Geometry: final body of the model. Coordinates: model frame, mm. Round coordinates to 2 decimals unless told otherwise and drop trailing zeros. Loops run counter-clockwise (first coordinate to the right, second up) from the corner with the lowest first, then second, coordinate; pieces in that order, holes last. Notation, with made-up numbers: (16.25, -27) -> (31.25, -27) arc R16 cw to (31.25, -8) -> close; hole circle Ø4 at (62.25, 22.25). An arc over 180 degrees is marked (long way). Answer in a Markdown table with one row per item.
```python
from build123d import *

# Parameters (mm, degrees)
SKETCH1_R               = 6.35
BOSS_EXTRUDE1_DEPTH     = 531
SKETCH2_R               = 5.5
BOSS_EXTRUDE2_DEPTH     = 2
BOSS_EXTRUDE3_START     = 2
SKETCH3_R               = 5.5
BOSS_EXTRUDE3_DEPTH     = 2
CUT_EXTRUDE1_DEPTH      = 536.075363851
CUT_EXTRUDE1_DEPTH_BACK = 536.075363851
SKETCH4_R               = 2.375


with BuildPart() as part:
    # Sketch1 → Boss-Extrude1 (new body)
    with BuildSketch(Plane.XY):
        Circle(SKETCH1_R)
    extrude(amount=BOSS_EXTRUDE1_DEPTH)

    # Sketch2 → Boss-Extrude2 (add)
    with BuildSketch(Plane.XY.offset(531)):
        Circle(SKETCH2_R)
    extrude(amount=BOSS_EXTRUDE2_DEPTH)

    # Sketch3 → Boss-Extrude3 (add)
    with BuildSketch(Plane(origin=(0, 0, 0), x_dir=(-1, 0, 0), z_dir=(0, 0, -1)).offset(BOSS_EXTRUDE3_START)):
        with Locations(Location((0, 0, 0), (0, 0, 180))):
            Circle(SKETCH3_R)
    extrude(amount=-BOSS_EXTRUDE3_DEPTH)

    # Sketch4 → Cut-Extrude1 (cut, two sides: drawn at the far end of the back side and taken through both)
    with BuildSketch(Plane(origin=(0, 0, -2), x_dir=(-1, 0, 0), z_dir=(0, 0, -1)).offset(-CUT_EXTRUDE1_DEPTH_BACK)):
        Circle(SKETCH4_R)
    extrude(amount=CUT_EXTRUDE1_DEPTH + CUT_EXTRUDE1_DEPTH_BACK, mode=Mode.SUBTRACT)


solid = part.part
```
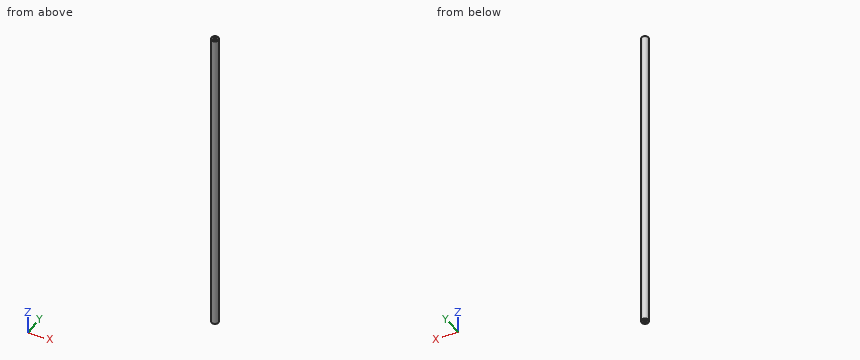
Item 1: Cut plane A-A (y = 0). Output: boundary loops of the cut face in (x, z) (3 decimals).
Answer:
| item | result |
|---|---|
| outline | (-6.35, 0) -> (-5.5, 0) -> (-5.5, -2) -> (-2.375, -2) -> (-2.375, 533) -> (-5.5, 533) -> (-5.5, 531) -> (-6.35, 531) -> close; (2.375, -2) -> (5.5, -2) -> (5.5, 0) -> (6.35, 0) -> (6.35, 531) -> (5.5, 531) -> (5.5, 533) -> (2.375, 533) -> close |
Item 2: Pin query (flat end, axial travel): pin 1 Ø1.5 at (y, z) = (3, 384) entering from +X; pin 2 Ø3 at (x, y) = (0, 0) entering from +Z. Return the tip coordinate at first contact, or that it passes through.
Answer:
| item | result |
|---|---|
| pin 1 | stops at x = 5.94 |
| pin 2 | passes through |
Item 3: Line query: probe 1 along Y at (x, z) = (0, 204.5) (3 decimals); probe 2 along X at (y, z) = (-0.5, 39.5); probe 3 along Z at (x, y) = (-1.75, -5.5). Output: solid intervals per line, ascending. Write a range as [from, to].
Answer:
| item | result |
|---|---|
| probe 1 | y = [-6.35, -2.375], [2.375, 6.35] |
| probe 2 | x = [-6.33, -2.32], [2.32, 6.33] |
| probe 3 | z = [0, 531] |
Item 4: Cut plane C-C (z = 34). Output: boundary loops of the cut face in (x, y) (3 decimals), then the cut area to 3 significant figures.
Answer:
| item | result |
|---|---|
| outline | circle Ø12.7 at (0, 0); hole circle Ø4.75 at (0, 0) |
| area | 109 mm² |
